Here's how the part is built. I have some questions about the finished solid (model axes, mm). Face numbers are marked on the shaded views. A direction names the side the tool comes from. Round coordinates to 2 decimals unless told otherwise and drop trailing zeros. Loops run counter-clockwise (first coordinate to the right, second up) from the corner with the lowest first, then second, coordinate; pieces in that order, holes last. Notation, with made-up numbers: M 42,5.5 L 80,5.5 A23 cw 80,20.5 Z; hole C 58,10.5 d11. An arc over 180 degrees is marked long. Answer as a JSON object with one key per item and string values.
from build123d import *

# Parameters (mm, degrees)
IZIM1_R                     = 7.5
Y_KSEKLIK_EKSTR_ZYON1_DEPTH = 5
IZIM6_R                     = 5
Y_KSEKLIK_EKSTR_ZYON5_DEPTH = 5
Y_KSEKLIK_EKSTR_ZYON6_DEPTH = 7
DAIRESEL_KAPLAMA2_COUNT     = 20
IZIM8_R                     = 7.5
Y_KSEKLIK_EKSTR_ZYON7_DEPTH = 1
IZIM9_R                     = 2.5
KES_EKSTR_ZYON2_DEPTH       = 21
IZIM10_R                    = 1.2
KES_EKSTR_ZYON3_DEPTH       = 21


with BuildPart() as part:
    # Çizim1 → Yükseklik-Ekstrüzyon1 (new body)
    with BuildSketch(Plane(origin=(0, 0, 0), x_dir=(1, 0, 0), z_dir=(0, 1, 0))):
        Circle(IZIM1_R)
    extrude(amount=Y_KSEKLIK_EKSTR_ZYON1_DEPTH)

    # Çizim6 → Yükseklik-Ekstrüzyon5 (add)
    with BuildSketch(Plane(origin=(0, 5, 0), x_dir=(1, 0, 0), z_dir=(0, 1, 0))):
        Circle(IZIM6_R)
    extrude(amount=Y_KSEKLIK_EKSTR_ZYON5_DEPTH)

    # Çizim7 → Yükseklik-Ekstrüzyon6 (add)
    with BuildSketch(Plane(origin=(0, 10, 0), x_dir=(1, 0, 0), z_dir=(0, 1, 0))):
        with BuildLine():
            Line((0, 6), (0, 5))
            ThreePointArc((0, 5), (0.223628846, 4.99499651), (0.446810123, 4.979996056))
            Line((0.446810123, 4.979996056), (0.446810123, 6))
            Line((0.446810123, 6), (0, 6))
        make_face()
        with BuildLine():
            ThreePointArc((-0.553189877, 4.969303871), (-0.277020438, 4.99232007), (0, 5))
            Line((0, 5), (0, 6))
            Line((0, 6), (-0.553189877, 6))
            Line((-0.553189877, 6), (-0.553189877, 4.969303871))
        make_face()
    y_kseklik_ekstr_zyon6 = extrude(amount=-Y_KSEKLIK_EKSTR_ZYON6_DEPTH)

    # Dairesel Kaplama2: Yükseklik-Ekstrüzyon6 ×20 about axis
    dairesel_kaplama2_axis = Axis((0, 0, 0), (0, 1, 0))
    for i in range(1, DAIRESEL_KAPLAMA2_COUNT):
        add(y_kseklik_ekstr_zyon6.rotate(dairesel_kaplama2_axis, i * 360 / DAIRESEL_KAPLAMA2_COUNT))

    # Çizim8 → Yükseklik-Ekstrüzyon7 (add)
    with BuildSketch(Plane(origin=(0, 10, 0), x_dir=(1, 0, 0), z_dir=(0, 1, 0))):
        Circle(IZIM8_R)
    extrude(amount=Y_KSEKLIK_EKSTR_ZYON7_DEPTH)

    # Çizim9 → Kes-Ekstrüzyon2 (cut)
    with BuildSketch(Plane(origin=(0, 11, 0), x_dir=(1, 0, 0), z_dir=(0, 1, 0))):
        Circle(IZIM9_R)
    extrude(amount=-KES_EKSTR_ZYON2_DEPTH, mode=Mode.SUBTRACT)

    # Çizim10 → Kes-Ekstrüzyon3 (cut)
    with BuildSketch(Plane(origin=(0, 0, 0), x_dir=(0, 0, -1), z_dir=(1, 0, 0))):
        with Locations((0, 2.361227205)):
            Circle(IZIM10_R)
    extrude(amount=-KES_EKSTR_ZYON3_DEPTH, mode=Mode.SUBTRACT)


solid = part.part
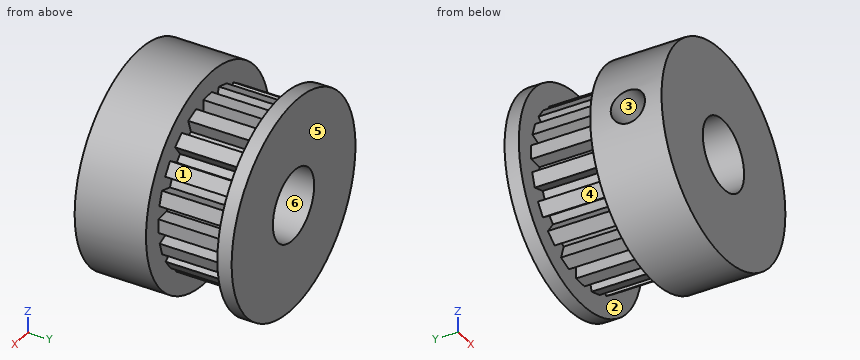
Item 1: I want a section at A-A on x = 0. List the corners of the cut face in (y, z) for me, plus the area to 3 significant figures.
Solution:
{"outline": "M 0,-7.5 L 5,-7.5 L 5,-6 L 10,-6 L 10,-7.5 L 11,-7.5 L 11,-2.5 L 0,-2.5 Z; M 0,2.5 L 11,2.5 L 11,7.5 L 10,7.5 L 10,6 L 5,6 L 5,7.5 L 0,7.5 Z", "area": "95.0 mm2"}
Item 2: We'd pull the mould along Z, two halves only. Please class the marked faces 4, 5 and 6: +Z half, -Z half, draft (parallel to the pull), parting line (faces both ways), or undercut.
Solution:
{"face 4": "-Z half", "face 5": "draft", "face 6": "undercut"}
Item 3: I want a section at B-B on z = 0. List the corners of the cut face in (x, y) for me, plus the area to 3 significant figures.
Solution:
{"outline": "M -7.5,0 L -2.5,0 L -2.5,1.16 L -7.5,1.16 Z; M -7.5,3.56 L -2.5,3.56 L -2.5,11 L -7.5,11 L -7.5,10 L -6,10 L -6,5 L -7.5,5 Z; M 2.5,0 L 7.5,0 L 7.5,5 L 6,5 L 6,10 L 7.5,10 L 7.5,11 L 2.5,11 Z", "area": "83.0 mm2"}
Item 4: For the marked faces 1, 2 and 3, which set-ups out of +Z, -Z, +X, -X, +Y, -Y let a thin tool reach every point of the face, with its end or its side?
Solution:
{"face 1": "+Z, +X", "face 2": "none", "face 3": "-X"}
Item 5: For P1, Ø0.5, axis at x = -5.5, y = 6.5, coming from the -Z side; P2, Ø2, axis at y = 7, z = -2, coming from the -X side; P3, Ø1.1, axis at y = 8, z = 5.5, coming from the +X side, each with a flat end and sliding along its axis, tell me the tip position at first contact or that it passes through.
Solution:
{"P1": "stops at z = -2.28", "P2": "stops at x = -5.88", "P3": "stops at x = 3.39"}
Item 6: I want a section at C-C on y = 4. List the corners of the cut face in (x, z) for me.
Solution:
{"outline": "C 0,0 d15; hole C 0,0 d5"}
Item 7: I want a section at D-D on x = -1.75. List the corners of the cut face in (y, z) for me.
Solution:
{"outline": "M 0,-7.29 L 5,-7.29 L 5,-5.74 L 10,-5.74 L 10,-7.29 L 11,-7.29 L 11,-1.79 L 0,-1.79 Z; M 0,1.79 L 11,1.79 L 11,7.29 L 10,7.29 L 10,5.74 L 5,5.74 L 5,7.29 L 0,7.29 Z"}
Item 8: If I drill on L1, parallel to Z at x = 4.5, y = 6.75; L2, parallel to Y at x = -3.4, z = 0; L3, parallel to Z at x = 0, y = 3.75, over which ranges is the centre line in solid material (lowest first)? Write a range as from..to.
Solution:
{"L1": "z = -3.95..-2.72, -2.18..2.18, 2.59..3.82", "L2": "y = 0..1.16, 3.56..11", "L3": "z = -7.5..-2.5, 2.5..7.5"}
